The drawing under review shows one solid part. Ordinate dimensions are in mm from its lowest x, y, z. A direction names the side the tool comes from. Give positions to 0.01 mm unless a question says otherwise; leave off trailing zeros. Order: outer loops, then holes, each group sorted by start corner. A loop starts at its lowest first (then second) coordinate and runs counter-clockwise, first axis right, second up. Notation, with made-up numbers: (55.5, 61.5) - (59.5, 61.5) arc R19 ccw to (59.5, 67.5) - close; hole circle Ø7 at (77, -23.75). An arc over 180 degrees is marked (long way). Write item = value, one per line. Start each with the question number.
1. For P1, Ø9, axis at x = 25.13, z = 27.5, coming from the +Y side; P2, Ø6, axis at x = 48, y = 5, coming from the +Z side, all flat-tipped, find the tip position at first contact; note any pin that passes through.
2. We need section B-B, the plane z = 27.5. Give the boundary of the cut face in (x, y), and give its area (3 significant figures).
3. We need section C-C, the plane y = 8.75. Give the boundary of the cut face in (x, z), and give its area (3 significant figures).
4. Mouldability with a two-part tool opening along Z and no side actions: class the marked faces 1, 2 and 3 as pulls with the +Z half, pulls with the -Z half, needs draft (parallel to the pull), parting line crosses it, or undercut.
5. We need section D-D, the plane y = 22. Give the boundary of the cut face in (x, z).
6. We need section A-A, the plane x = 43. Give the boundary of the cut face in (y, z).
7. Machinability: for the marked faces 4 and 5, which of the approach directions +Z, -Z, +X, -X, +Y, -Y give a long, thin tool a straight path to every point of the face, cutting with its end or side? Answer none if there is none.
8. Wall thickness on probe 1 along X at (y, z) = (18, 13); probe 2 along X at (y, z) = (4.75, 10); probe 3 along Z at (x, y) = (67.5, 7.75): over which ranges is each line inside the solid? List them lowest first.
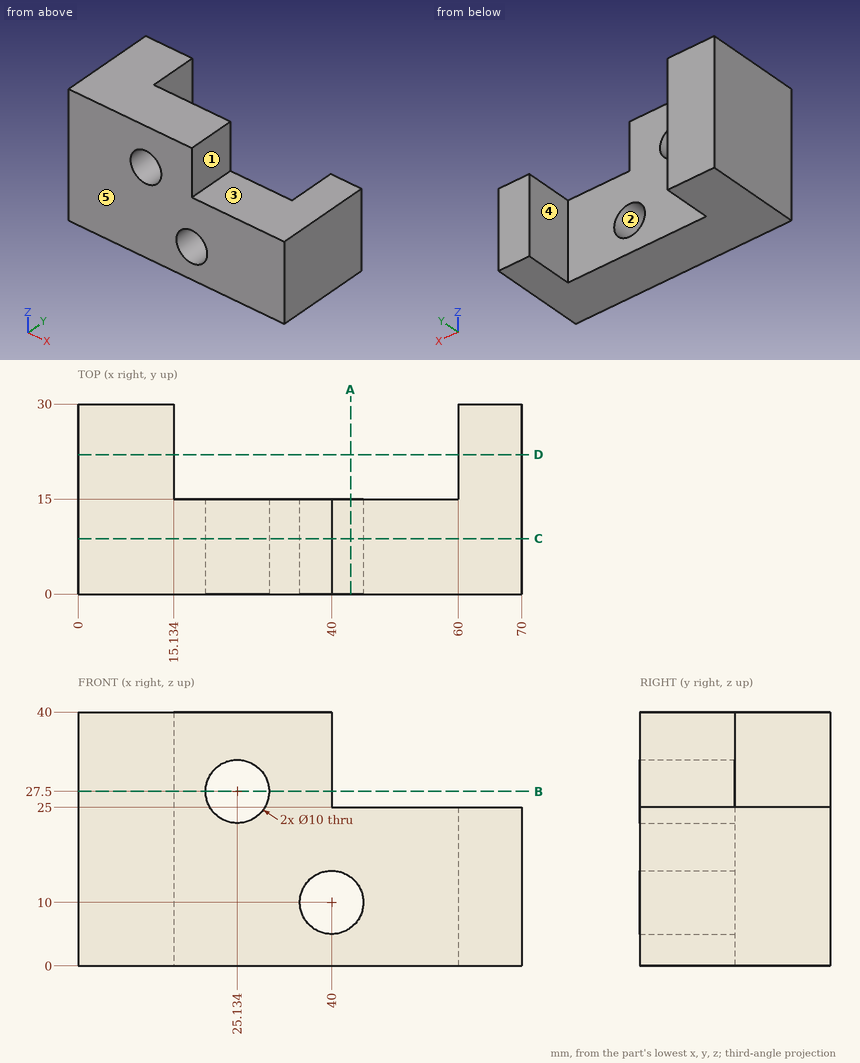
Model answer:
q1.P1 = through
q1.P2 = 25
q2.outline = (0, 0) - (20.13, 0) - (20.13, 15) - (15.13, 15) - (15.13, 30) - (0, 30) - close; (30.13, 0) - (40, 0) - (40, 15) - (30.13, 15) - close
q2.area = 677 mm2
q3.outline = (0, 0) - (70, 0) - (70, 25) - (40, 25) - (40, 40) - (0, 40) - close; hole circle Ø10 at (25.13, 27.5); hole circle Ø10 at (40, 10)
q3.area = 2,190 mm2
q4.face_1 = needs draft
q4.face_2 = undercut
q4.face_3 = pulls with the +Z half
q5.outline = (0, 0) - (15.13, 0) - (15.13, 40) - (0, 40) - close; (60, 0) - (70, 0) - (70, 25) - (60, 25) - close
q6.outline = (0, 0) - (15, 0) - (15, 6) - (0, 6) - close; (0, 14) - (15, 14) - (15, 25) - (0, 25) - close
q7.face_4 = +Z, -Z, +Y
q7.face_5 = +Z, -Z, +X, -X, -Y
q8.probe_1 = 0 to 15.13, 60 to 70
q8.probe_2 = 0 to 35, 45 to 70
q8.probe_3 = 0 to 25
